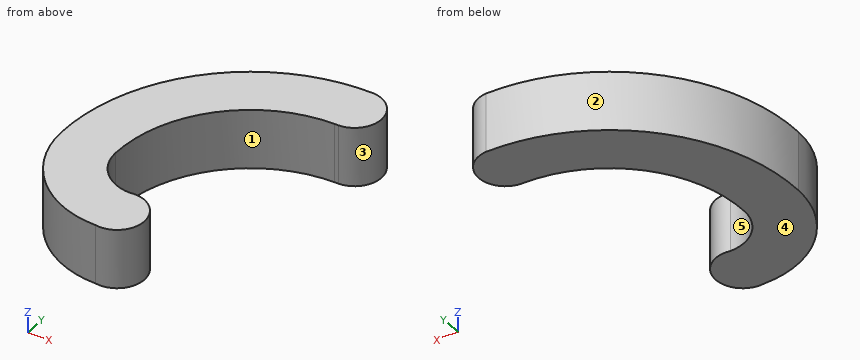
from build123d import *

# Parameters (mm, degrees)
F1_DEPTH = 12.7


with BuildPart() as f1:
    # F0 (on Top) → F1 (new body)
    with BuildSketch(Plane.XY):
        with BuildLine():
            ThreePointArc((-0.856272, 28.302937), (-0.428185, 28.312649), (0, 28.315887))
            ThreePointArc((0, 28.315887), (5.32199, 33.984497), (0, 39.653108))
            ThreePointArc((0, 39.653108), (-28.038981, 28.038981), (-39.653108, 0))
            ThreePointArc((-39.653108, 0), (-33.749679, -14.1228), (-19.551708, -19.843075))
            ThreePointArc((-19.551708, -19.843075), (-12.931084, -14.028775), (-19.797987, -8.507508))
            ThreePointArc((-19.797987, -8.507508), (-25.820421, -6.019392), (-28.315887, 0))
            ThreePointArc((-28.315887, 0), (-20.322839, 19.717294), (-0.856272, 28.302937))
        make_face()
    extrude(amount=F1_DEPTH)


solid = f1.part
Input: part model. Units: mm. Frame: model coordinates. Face numbers are marked on the shaded views. A direction names the side the tool comes from. Give positions to 0.01 mm unless a question says otherwise; leave off trailing zeros. Loops run counter-clockwise (first coordinate to the right, second up) from the corner with the lowest first, then second, coordinate; pieces in that order, holes last. Notation, with made-up numbers: (54, -40) -> (99, -40) arc R21 cw to (99, -30) -> close; hole circle Ø1 at (67.25, 13). An arc over 180 degrees is marked (long way). Answer as a JSON object with one key per item and string values. Group by question number.
Item 1: Cut plane C-C, the plane y = 12. Return the cut outline in (x, z), and give its area (3 significant figures).
Item 2: Pin query (flat end, axial travel): P1, Ø1.5, axis at x = -30.5, z = 5, coming from the -Y side; P2, Ø6, axis at x = -23.5, y = 26, coming from the -Z side; P3, Ø5, axis at y = 8, z = 4.5, coming from the -X side; P4, Ø2, axis at y = 9.5, z = 4.5, coming from the -X side. Return the tip coordinate at first contact, or that it passes through.
Item 3: Reachability of the marked faces 1 and 2 from +Z, -Z, +X, -X, +Y, -Y: full face, straight path, thin tool, end or side. Return the list, or none.
Item 4: Pull-direction query (Y, two-part tool) for the marked faces 3, 4 and 5; classes: released by +Y, released by -Y, zero draft, split by the parting line, or undercut.
Item 5: Cut plane D-D, the plane x = -31. Return the cut outline in (y, z), and give its area (3 significant figures).
Item 6: Line query: probe 1 along Y at (x, z) = (-15.5, 8.5); probe 2 along Y at (x, z) = (-25, 8.25); probe 3 along X at (y, z) = (19.5, 7.75). Output: solid intervals per line, ascending.
Item 7: Cut plane A-A, the plane x = -14. Return the cut outline in (y, z), and give its area (3 significant figures).
Item 8: Cut plane B-B, the plane z = 11.25. Return the cut outline in (x, y), and give its area (3 significant figures).
Checks:
{
 "1": {"outline": "(-37.79, 0) -> (-25.65, 0) -> (-25.65, 12.7) -> (-37.79, 12.7) -> close", "area": "154 mm²"},
 "2": {"P1": "stops at y = -17.17", "P2": "stops at z = 0", "P3": "stops at x = -39.27", "P4": "stops at x = -38.73"},
 "3": {"face 1": "+Z, -Z, +X", "face 2": "+Z, -Z, -X, +Y"},
 "4": {"face 3": "split by the parting line", "face 4": "zero draft", "face 5": "undercut"},
 "5": {"outline": "(-16.39, 0) -> (24.73, 0) -> (24.73, 12.7) -> (-16.39, 12.7) -> close", "area": "522 mm²"},
 "6": {"probe 1": "y = -18.95 to -9.36, 23.7 to 36.5", "probe 2": "y = -19.15 to -6.74, 13.3 to 30.78", "probe 3": "x = -34.53 to -20.53"},
 "7": {"outline": "(-17.5, 0) -> (-10.81, 0) -> (-10.81, 12.7) -> (-17.5, 12.7) -> close; (24.61, 0) -> (37.1, 0) -> (37.1, 12.7) -> (24.61, 12.7) -> close", "area": "243 mm²"},
 "8": {"outline": "(-39.65, 0) arc R19.84 ccw to (-19.55, -19.84) arc R5.75 ccw (long way) to (-19.8, -8.51) arc R8.51 cw to (-28.32, 0) arc R28.32 cw to (-0.86, 28.3) arc R28.32 cw to (0, 28.32) arc R5.68 ccw to (0, 39.65) arc R39.65 ccw to start", "area": "969 mm²"}
}
